```python
from build123d import *

# Parameters (mm, degrees)
SKETCH1_W           = 38
SKETCH1_H           = 32
BOSS_EXTRUDE1_DEPTH = 13
SKETCH2_R           = 2
CUT_EXTRUDE1_DEPTH  = 8
SKETCH3_R           = 4
CUT_EXTRUDE2_DEPTH  = 44.231932642


with BuildPart() as part:
    # Sketch1 → Boss-Extrude1 (new body)
    with BuildSketch(Plane(origin=(0, 0, 0), x_dir=(1, 0, 0), z_dir=(0, 1, 0))):
        Rectangle(SKETCH1_W, SKETCH1_H)
    extrude(amount=BOSS_EXTRUDE1_DEPTH)

    # Sketch2 → Cut-Extrude1 (cut)
    with BuildSketch(Plane(origin=(0, 13, 0), x_dir=(1, 0, 0), z_dir=(0, 1, 0))):
        with Locations(Location((8.5, 8.5, 0), (0, 0, 270))):
            Circle(SKETCH2_R)
        with Locations(Location((-8.5, 8.5, 0), (0, 0, 90))):
            Circle(SKETCH2_R)
        with Locations(Location((-8.5, -8.5, 0), (0, 0, 270))):
            Circle(SKETCH2_R)
        with Locations(Location((8.5, -8.5, 0), (0, 0, 90))):
            Circle(SKETCH2_R)
    extrude(amount=-CUT_EXTRUDE1_DEPTH, mode=Mode.SUBTRACT)

    # Sketch3 → Cut-Extrude2 (cut, through all)
    with BuildSketch(Plane(origin=(19, 0, 0), x_dir=(0, 0, -1), z_dir=(1, 0, 0))):
        with Locations((0, 6.5)):
            Circle(SKETCH3_R)
    extrude(amount=-CUT_EXTRUDE2_DEPTH, mode=Mode.SUBTRACT)


solid = part.part
```
Here's how the part is built. I have some questions about the finished solid (model axes, mm). A direction names the side the tool comes from. Coordinates: 2 decimals unless noted, no trailing zeros. Order: outer loops, then holes, each group sorted by start corner. A loop starts at its lowest first (then second) coordinate and runs counter-clockwise, first axis right, second up. Notation, with made-up numbers: M -15.5,-26.75 L 21.5,-26.75 A22 cw 21.5,1.25 Z; hole C -10.75,42 d10. An arc over 180 degrees is marked long. Answer as a JSON object with one key per item and string values. Group by question number.
(1) Suppose I cut it at C-C, the plane x = -3. Please give me the cut outline in (y, z), then the cut area to 3 significant figures.
(2) If we mould it in two halves opening along Z, with no side actions, what happens to faces 3 (the face through (0, 6, 16)), 4 (the face through (-19, 5, 4)), 5 (the face through (8, 5, 9))? For each: released by +Z, released by -Z, zero draft, split by the parting line, or undercut.
(3) Suppose I cut it at B-B, the plane y = 6.5. Please give me the cut outline in (x, z), then the cut area to 3 significant figures.
(4) Suppose I cut it at A-A, the plane z = 0. Please give me the cut outline in (x, y).
(5) For pin 1 (1.2 mm diameter, centred on x = 8.5, z = -8.5, fed in from +Y); pin 2 (3 mm diameter, centred on x = -9.5, z = 9.5, fed in from +Y), each with a flat end and sliding along its axis, tell me the tip position at first contact or that it passes through.
(6) I need wall thicknesses on probe 1 along X at (y, z) = (8, -8.5); probe 2 along Y at (x, z) = (-5, 0); probe 3 along Z at (x, y) = (9.5, 11.25). Which ranges of each line are inside material? Lowest first, please.
(7) Which directions (+Z, -Z, +X, -X, +Y, -Y) give clear straight access to the entire face, cutting with the end or side of a thin tool? Please do faces 1 (the face through (-8, 5, 8)), 2 (the face through (0.266, 2.595, 0.867)).
(8) Suppose I cut it at D-D, the plane z = 8.5. Please give me the cut outline in (x, y).
Values found:
{
 "1": {"outline": "M 0,-16 L 13,-16 L 13,16 L 0,16 Z; hole C 6.5,0 d8", "area": "366 mm^2"},
 "2": {"face 3": "released by +Z", "face 4": "zero draft", "face 5": "undercut"},
 "3": {"outline": "M -19,-16 L 19,-16 L 19,-4 L -19,-4 Z; M -19,4 L 19,4 L 19,16 L -19,16 Z; hole C -8.5,-8.5 d4; hole C -8.5,8.5 d4; hole C 8.5,-8.5 d4; hole C 8.5,8.5 d4", "area": "862 mm^2"},
 "4": {"outline": "M -19,0 L 19,0 L 19,2.5 L -19,2.5 Z; M -19,10.5 L 19,10.5 L 19,13 L -19,13 Z"},
 "5": {"pin 1": "stops at y = 5", "pin 2": "stops at y = 13"},
 "6": {"probe 1": "x = -19 to -10.5, -6.5 to 6.5, 10.5 to 19", "probe 2": "y = 0 to 2.5, 10.5 to 13", "probe 3": "z = -16 to -10.23, -6.77 to 6.77, 10.23 to 16"},
 "7": {"face 1": "+Y", "face 2": "+X, -X"},
 "8": {"outline": "M -19,0 L 19,0 L 19,13 L 10.5,13 L 10.5,5 L 6.5,5 L 6.5,13 L -6.5,13 L -6.5,5 L -10.5,5 L -10.5,13 L -19,13 Z"}
}
